Geometry check sheet. Reference: the model listing, model coordinates, mm. Coordinates: 2 decimals unless noted, no trailing zeros. Write each loop counter-clockwise with the first axis right and the second up, starting at its lowest first coordinate (ties: lowest second). Pieces come first, ordered by that corner, then holes. Notation, with made-up numbers: (-14, -23) -> (21, -23) arc R19 ccw to (21, -13) -> close; hole circle Ø7 at (-8.75, -26). An arc over 180 degrees is marked (long way). Answer in a Markdown table with one row per item. Add a question column.
1. Scan lines: L1, parallel to X at y = 55, z = 24; L2, parallel to Y at x = -644, z = 12. Record each from-to range of solid material in increasing order. Write a range as from..to.
2. Depth check by flat-ended pin: P1, Ø4, axis at x = -349.5, z = -21.5, coming from the +Y side. Enter the tip coordinate at first touch or a pass-through.
3. Cross-section at A-A on z = -26. Record the cut outline in (x, y).
4. Mould release check, pull along X, two halves, no side actions. Record for faces 1 (the flat face through (-1316.99, 31, 1)), 2 (the flat face through (1047, 25, 38.1)), 3 (the flat face through (-18, 50.8, -1)): pulls with the +X half, pulls with the -X half, needs draft (parallel to the pull), parting line crosses it, or undercut.
5. Cross-section at B-B on x = -123.5. Record the cut outline in (y, z).
```python
from build123d import *

# Parameters (mm, degrees)
SKETCH1_W           = 2633.98
SKETCH1_H           = 76.2
BOSS_EXTRUDE1_DEPTH = 50.8
SKETCH2_W           = 19.05
SKETCH2_H           = 63.5
CUT_REVOLVE4_ANGLE  = 103
SKETCH3_W           = 21.59
SKETCH3_H           = 76.2
BOSS_EXTRUDE2_DEPTH = 12.7


with BuildPart() as part:
    # Sketch1 → Boss-Extrude1 (new body)
    with BuildSketch(Plane(origin=(0, 0, 0), x_dir=(1, 0, 0), z_dir=(0, 1, 0))):
        Rectangle(SKETCH1_W, SKETCH1_H)
    extrude(amount=BOSS_EXTRUDE1_DEPTH)

    # Sketch2 → Cut-Revolve4 (revolve, cut)
    with BuildSketch(Plane(origin=(0, 50.8, 0), x_dir=(1, 0, 0), z_dir=(0, 1, 0))):
        with Locations((-962.025, -69.85)):
            Rectangle(SKETCH2_W, SKETCH2_H)
        with Locations((-1133.475, -69.85)):
            Rectangle(SKETCH2_W, SKETCH2_H)
        with Locations((962.025, -69.85)):
            Rectangle(SKETCH2_W, SKETCH2_H)
        with Locations((1133.475, -69.85)):
            Rectangle(SKETCH2_W, SKETCH2_H)
    revolve(axis=Axis((-1316.99, 50.8, 38.1), (1, 0, 0)), revolution_arc=CUT_REVOLVE4_ANGLE, mode=Mode.SUBTRACT)

    # Sketch3 → Boss-Extrude2 (add)
    with BuildSketch(Plane(origin=(0, 50.8, 0), x_dir=(1, 0, 0), z_dir=(0, 1, 0))):
        with Locations((-1306.195, 0)):
            Rectangle(SKETCH3_W, SKETCH3_H)
        with Locations((1306.195, 0)):
            Rectangle(SKETCH3_W, SKETCH3_H)
    extrude(amount=BOSS_EXTRUDE2_DEPTH)


solid = part.part
```
Results found:
| question | item | result |
|---|---|---|
| 1 | L1 | x = -1316.99..-1295.4, 1295.4..1316.99 |
| 1 | L2 | y = 0..50.8 |
| 2 | P1 | stops at y = 50.8 |
| 3 | outline | (-1316.99, 0) -> (1316.99, 0) -> (1316.99, 63.5) -> (1295.4, 63.5) -> (1295.4, 50.8) -> (-1295.4, 50.8) -> (-1295.4, 63.5) -> (-1316.99, 63.5) -> close |
| 4 | face 1 | pulls with the -X half |
| 4 | face 2 | needs draft |
| 4 | face 3 | undercut |
| 5 | outline | (0, -38.1) -> (50.8, -38.1) -> (50.8, 38.1) -> (0, 38.1) -> close |
